Input: part model. Units: mm. Frame: model coordinates. A direction names the side the tool comes from. Give positions to 0.01 mm unless a question says otherwise; leave off trailing zeros. Write each loop counter-clockwise with the first axis right and the second up, starting at its lowest first coordinate (ties: lowest second). Pieces come first, ordered by that corner, then holes. Notation, with made-up numbers: (9.25, 88.5) - (49.25, 88.5) arc R10 cw to (49.25, 103.5) - close; hole circle Ø11 at (-33.75, 6.5). An arc over 180 degrees is marked (long way). Answer as CSV lines item,"result".
```python
from build123d import *

# Parameters (mm, degrees)
F2_R     = 1.25
F3_DEPTH = 15
F5_DEPTH = 30.001


with BuildPart() as f1:
    # F0 (on Front) → F1 (revolve)
    with BuildSketch(Plane.XZ):
        Polygon((34.5, 30), (26.5, 30), (26.5, 0), (38.5, 0), (38.5, 12), align=None)
    revolve(axis=Axis((0, 0, 21.473579), (0, 0, 1)))

    # F2 (on face) → F3 (cut)
    with BuildSketch(Plane(origin=(0, 0, 0), x_dir=(1, 0, 0), z_dir=(0, 0, -1))):
        with Locations((-28, -6)):
            Circle(F2_R)
        with Locations((28, 6)):
            Circle(F2_R)
    extrude(amount=-F3_DEPTH, mode=Mode.SUBTRACT)

    # F4 (on face) → F5 (cut, through all)
    with BuildSketch(Plane(origin=(0, 0, 0), x_dir=(1, 0, 0), z_dir=(0, 0, -1))):
        with BuildLine():
            Line((-48.065083, -10.141205), (-30.5, 0))
            ThreePointArc((-30.5, 0), (-26.749196, 14.653687), (-16.419309, 25.703235))
            Line((-16.419309, 25.703235), (-33.739817, 35.703235))
            ThreePointArc((-33.739817, 35.703235), (-46.88751, 14.6512), (-48.065083, -10.141205))
        make_face()
        with BuildLine():
            Line((-30.469309, -1.367921), (-47.789817, -11.367921))
            ThreePointArc((-47.789817, -11.367921), (-36.132066, -33.280175), (-15.25, -46.696186))
            Line((-15.25, -46.696186), (-15.25, -26.413775))
            ThreePointArc((-15.25, -26.413775), (-26.065063, -15.838639), (-30.469309, -1.367921))
        make_face()
        with BuildLine():
            Line((-14.05, -27.071156), (-14.05, -47.071156))
            ThreePointArc((-14.05, -47.071156), (10.755444, -47.931375), (32.815083, -36.55498))
            Line((32.815083, -36.55498), (15.25, -26.413775))
            ThreePointArc((15.25, -26.413775), (0.684133, -30.492326), (-14.05, -27.071156))
        make_face()
        with BuildLine():
            Line((16.419309, -25.703235), (33.739817, -35.703235))
            ThreePointArc((33.739817, -35.703235), (46.88751, -14.6512), (48.065083, 10.141205))
            Line((48.065083, 10.141205), (30.5, 0))
            ThreePointArc((30.5, 0), (26.749196, -14.653687), (16.419309, -25.703235))
        make_face()
        with BuildLine():
            Line((30.469309, 1.367921), (47.789817, 11.367921))
            ThreePointArc((47.789817, 11.367921), (36.132066, 33.280175), (15.25, 46.696186))
            Line((15.25, 46.696186), (15.25, 26.413775))
            ThreePointArc((15.25, 26.413775), (26.065063, 15.838639), (30.469309, 1.367921))
        make_face()
        with BuildLine():
            Line((14.05, 27.071156), (14.05, 47.071156))
            ThreePointArc((14.05, 47.071156), (-10.755444, 47.931375), (-32.815083, 36.55498))
            Line((-32.815083, 36.55498), (-15.25, 26.413775))
            ThreePointArc((-15.25, 26.413775), (-0.684133, 30.492326), (14.05, 27.071156))
        make_face()
    extrude(amount=-F5_DEPTH, mode=Mode.SUBTRACT)


solid = f1.part
```
Item 1: Ray query, line 1 (Y direction, x = -23, z = 10); line 2 (X direction, y = -4, z = 9.5); line 3 (X direction, y = 6, z = 7.5). Return the intervals inside material, ascending. Write a range as from..to.
The answers:
line 1,"-30.87..-29.5, -20.03..-13.16, 13.16..20.03"
line 2,"-30.24..-26.2, 26.2..30.24, 35.03..37.43"
line 3,"-29.9..-29.25, -26.75..-25.81, 25.81..29.9"
Item 2: Cut plane A-A on x = 0. Return the cut outline in (y, z), plus the area to 3 significant figures.
The answers:
outline,"(-30.5, 0) - (-26.5, 0) - (-26.5, 30) - (-30.5, 30) - close; (26.5, 0) - (30.5, 0) - (30.5, 30) - (26.5, 30) - close"
area,"240 mm²"
Item 3: Cut plane D-D on x = -18. Return the cut outline in (y, z), plus the area to 3 significant figures.
The answers:
outline,"(-28, 0) - (-26.62, 0) - (-26.62, 30) - (-28, 30) - close; (-24.62, 0) - (-19.45, 0) - (-19.45, 30) - (-24.62, 30) - close; (19.45, 0) - (24.62, 0) - (24.62, 30) - (19.45, 30) - close"
area,"352 mm²"
Item 4: Cut plane B-B on z = 11. Return the cut outline in (x, y), plus the area to 3 significant figures.
The answers:
outline,"(-38.24, 4.47) - (-30.5, 0) arc R30.5 ccw to (-16.42, -25.7) - (-24.02, -30.09) arc R38.5 ccw to (-22.99, -30.88) - (-15.25, -26.41) arc R30.5 ccw to (14.05, -27.07) - (14.05, -35.84) arc R38.5 ccw to (15.25, -35.35) - (15.25, -26.41) arc R30.5 ccw to (30.47, -1.37) - (38.07, -5.75) arc R38.5 ccw to (38.24, -4.47) - (30.5, 0) arc R30.5 ccw to (16.42, 25.7) - (24.02, 30.09) arc R38.5 ccw to (22.99, 30.88) - (15.25, 26.41) arc R30.5 ccw to (-14.05, 27.07) - (-14.05, 35.84) arc R38.5 ccw to (-15.25, 35.35) - (-15.25, 26.41) arc R30.5 ccw to (-30.47, 1.37) - (-38.07, 5.75) arc R38.5 ccw to start; hole circle Ø2.5 at (-28, 6); hole circle Ø53 at (0, 0); hole circle Ø2.5 at (28, -6)"
area,"770 mm²"
Item 5: Contact query for flat-ended pins moving along their axis: pin 1 (8 mm diameter, centred on x = 4.5, z = 11.5, fed in from -Y); pin 2 (3 mm diameter, centred on x = 23, z = 25, fed in from +Y); pin 3 (3 mm diameter, centred on x = -1, z = 5, fed in from +Y). Output: stop coordinate, or through.
The answers:
pin 1,"y = -30.5"
pin 2,"y = 21.63"
pin 3,"y = 30.5"
Item 6: Cut plane C-C on y = -14. Return the cut outline in (x, z), plus the area to 3 significant figures.
The answers:
outline,"(-27.1, 0) - (-22.5, 0) - (-22.5, 30) - (-27.1, 30) - close; (22.5, 0) - (27.1, 0) - (27.1, 30) - (22.5, 30) - close"
area,"276 mm²"
Item 7: Reachability of faces 4 (the face through (28.577, -4.891, 7.395)), 5 (the face through (15.25, -30, 15)), 6 (the face through (20.17, 27.87, 14.79)), 7 (the face through (-18, -28, 15)) from +Z, -Z, +X, -X, +Y, -Y: full face, straight path, thin tool, end or side. Return the list, or none.
The answers:
face 4,"-Z"
face 5,"+Z, -Z, +X, -Y"
face 6,"+Z, -Z, +X"
face 7,"+Z, -Z, -Y"
Item 8: Mould query, pull axis Y, two halves, no side actions, for faces 1 (the face through (-15.25, 30, 15)), 2 (the face through (33.564, -1.769, 14.79)), 3 (the face through (26.85, 14.47, 14.79)). Classes: +Y half, -Y half, draft (parallel to the pull), parting line (faces both ways), or undercut.
The answers:
face 1,"draft"
face 2,"+Y half"
face 3,"undercut"
